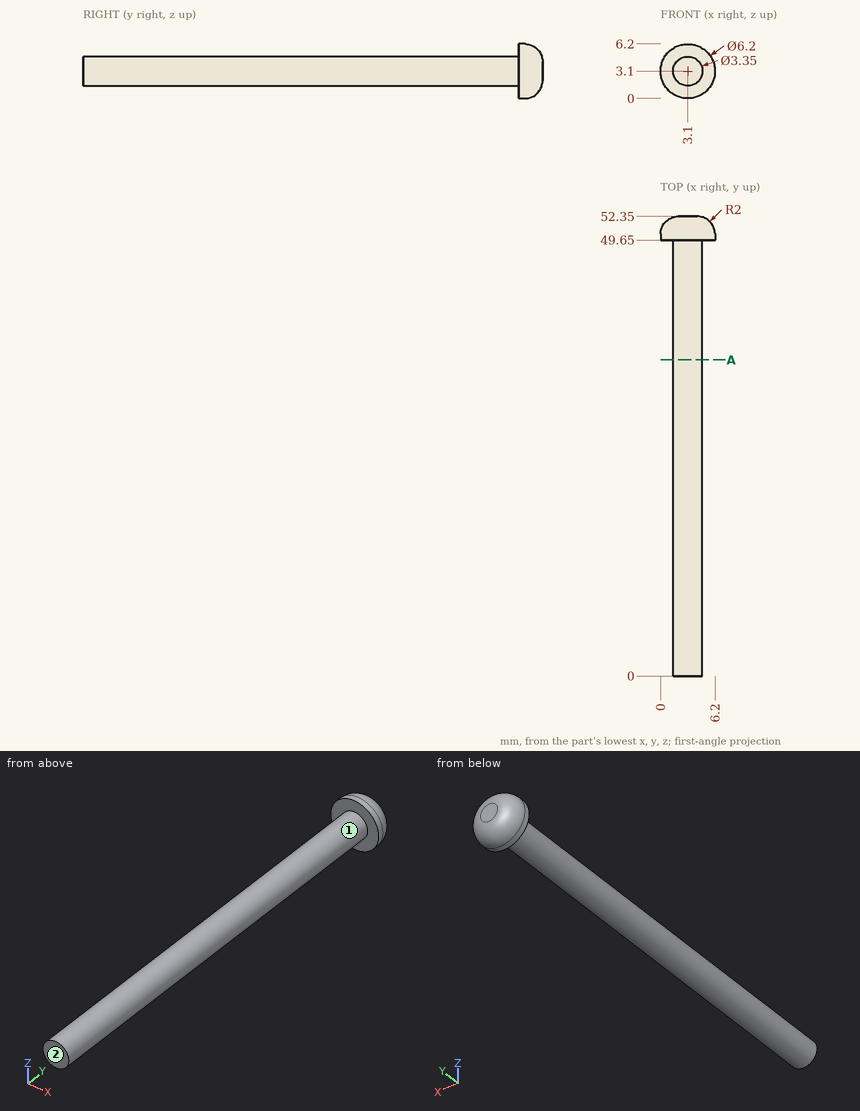
Design review of the part shown in the three views and the two pictorial views. Dimensions are in mm from the part's minimum x, y and z. A direction names the side the tool comes from. Round coordinates to 2 decimals unless told otherwise and drop trailing zeros. Order: outer loops, then holes, each group sorted by start corner. A loop starts at its lowest first (then second) coordinate and runs counter-clockwise, first axis right, second up.
(1) Wall thickness on L1, parallel to X at y = 41, z = 3.25; L2, parallel to Y at x = 4.75, z = 1.75; L3, parallel to Y at x = 1.25, z = 4.75: over which ranges is each line inside the solid? List them lowest first.
Working result:
L1: x = 1.43 to 4.77
L2: y = 49.65 to 52.06
L3: y = 49.65 to 51.8
(2) Take a section at A-A, the plane y = 36. State the section outline as (x, z) points (3 decimals), plus the area to 3 significant figures.
Working result:
outline: circle Ø3.35 at (3.1, 3.1)
area: 8.81 mm2
(3) For P1, Ø3, axis at y = 12, z = 3, coming from the +X side (3 decimals), flat-tipped, find the tip position at first contact; note if it passes through.
Working result:
P1: stops at x = 4.775
(4) Tool access review of the marked faces 1 and 2: name each direction out of +Z, -Z, +X, -X, +Y, -Y from which nothing blocks a thin tool from reaching the whole face with its end or side.
Working result:
face 1: -Y
face 2: +Z, -Z, +X, -X, -Y
